Autodesk Fusion 360 part; units mm, degrees
sketch "Sketch1" plane through (0, 0, 0) normal (0, 0, 1) x (1, 0, 0)
  circle A0 centre (0, 0) radius 7.55
  circle A1 centre (0, 0) radius 10.55
  dimension "d1" = 3
  dimension "d2" = 15.1
extrude "Extrude1" add sketch "Sketch1" along normal blind 10
extrude "Extrude2" add sketch "Sketch1" against normal blind 2 contours A0 | A1
fillet "Fillet1" radius 3 1 edges at (-9.8361, 3.815, -2)
CAD build for the part. Positions are in the model's coordinates, mm. Coordinates: 2 decimals unless noted, no trailing zeros. Order: outer loops, then holes, each group sorted by start corner. A loop starts at its lowest first (then second) coordinate and runs counter-clockwise, first axis right, second up. Notation, with made-up numbers: (-15.75, 42.5) - (-11.75, 42.5) arc R26 ccw to (-11.75, 72.5) - close; hole circle Ø5 at (82, -1). An arc over 180 degrees is marked (long way). Answer in a Markdown table with one row per item.
1. Pull direction Y, two halves, no side cores. Call faces 1 (the face through (10.063, -3.169, 5.437)), 2 (the face through (0, 0, -2)), 3 (the face through (0, 0, 0)), 4 (the face through (-1.64, 7.37, 4.93)): +Y half, -Y half, draft (parallel to the pull), parting line (faces both ways), or undercut.
Answer:
| item | result |
|---|---|
| face 1 | parting line |
| face 2 | draft |
| face 3 | undercut |
| face 4 | undercut |
2. Slice it at A-A, the plane z = 2.25. List the corners of the cut face in (x, y).
Answer:
| item | result |
|---|---|
| outline | circle Ø21.1 at (0, 0); hole circle Ø15.1 at (0, 0) |
3. Flat gauge pins, fed straight in: P1, Ø1, axis at x = 3.5, y = -3, coming from the +Z side; P2, Ø2, axis at y = -5.5, z = 4.5, coming from the -X side; P3, Ø5, axis at x = 6, z = 2.5, coming from the -Y side. Where does each tip first touch, or does it go through?
Answer:
| item | result |
|---|---|
| P1 | z = 0 |
| P2 | x = -9.54 |
| P3 | y = -9.95 |
4. Drill centre lines: L1, parallel to Y at x = 0, z = 6; L2, parallel to Y at x = -3.75, z = 3; L3, parallel to X at y = 5.5, z = 9.5. Where is each one in solid material? Low to high. Write a range as from..to.
Answer:
| item | result |
|---|---|
| L1 | -10.55..-7.55, 7.55..10.55 |
| L2 | -9.86..-6.55, 6.55..9.86 |
| L3 | -9..-5.17, 5.17..9 |
